Geometry check sheet. Reference: the model listing, model coordinates, mm. Give positions to 0.01 mm unless a question says otherwise; leave off trailing zeros. Loops run counter-clockwise (first coordinate to the right, second up) from the corner with the lowest first, then second, coordinate; pieces in that order, holes last. Notation, with made-up numbers: (83, -18.5) -> (124, -18.5) arc R25 ccw to (124, 16.5) -> close; hole circle Ø1 at (86, 41). An arc over 180 degrees is marked (long way). One line per item, written item: value. Start each with the question number.
(1) Sectioned sample at C-C, the plane z = -16. Record the cut outline in (x, y).
(2) Scan lines: line 1 along X through (y, z) = (-1.8, -15.5); line 2 along Z through (x, y) = (17, -0.85) (1 decimal); line 3 along X through (y, z) = (-1.05, 24). Record each from-to range of solid material in increasing order. Write a range as from..to.
(3) Sectioned sample at B-B, the plane x = 6.5. Record the cut outline in (y, z) (1 decimal).
(4) Gauge pin test, flat end, axial feed: pin 1 Ø5 at (x, z) = (-14, 20) entering from -Y. Record the tip position at first contact, or that the pin passes through.
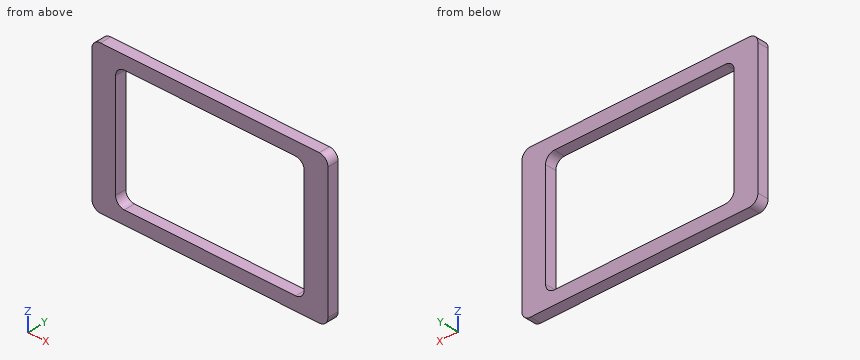
from build123d import *

# Parameters (mm, degrees)
F1_DEPTH = 4


with BuildPart() as f1:
    # F0 (on Front) → F1 (new body)
    with BuildSketch(Plane.XZ):
        with BuildLine():
            Line((0, 26.9875), (-39.7125, 26.9875))
            ThreePointArc((-39.7125, 26.9875), (-41.939886, 26.064886), (-42.8625, 23.8375))
            Line((-42.8625, 23.8375), (-42.8625, 0))
            Line((-42.8625, 0), (-34.25, 0))
            Line((-34.25, 0), (-34.25, 18.95))
            ThreePointArc((-34.25, 18.95), (-33.320064, 21.195064), (-31.075, 22.125))
            Line((-31.075, 22.125), (0, 22.125))
            Line((0, 22.125), (0, 26.9875))
        make_face()
        with BuildLine():
            Line((39.7125, 26.9875), (0, 26.9875))
            Line((0, 26.9875), (0, 22.125))
            Line((0, 22.125), (31.075, 22.125))
            ThreePointArc((31.075, 22.125), (33.320064, 21.195064), (34.25, 18.95))
            Line((34.25, 18.95), (34.25, -18.95))
            ThreePointArc((34.25, -18.95), (33.320064, -21.195064), (31.075, -22.125))
            Line((31.075, -22.125), (-31.075, -22.125))
            ThreePointArc((-31.075, -22.125), (-33.320064, -21.195064), (-34.25, -18.95))
            Line((-34.25, -18.95), (-34.25, 0))
            Line((-34.25, 0), (-42.8625, 0))
            Line((-42.8625, 0), (-42.8625, -23.8375))
            ThreePointArc((-42.8625, -23.8375), (-41.939886, -26.064886), (-39.7125, -26.9875))
            Line((-39.7125, -26.9875), (39.7125, -26.9875))
            ThreePointArc((39.7125, -26.9875), (41.939886, -26.064886), (42.8625, -23.8375))
            Line((42.8625, -23.8375), (42.8625, 23.8375))
            ThreePointArc((42.8625, 23.8375), (41.939886, 26.064886), (39.7125, 26.9875))
        make_face()
    extrude(amount=F1_DEPTH)


solid = f1.part
Calculated:
1. outline: (-42.86, -4) -> (-34.25, -4) -> (-34.25, 0) -> (-42.86, 0) -> close; (34.25, -4) -> (42.86, -4) -> (42.86, 0) -> (34.25, 0) -> close
2. line 1: x = -42.86..-34.25, 34.25..42.86
2. line 2: z = -27..-22.1, 22.1..27
2. line 3: x = -42.86..42.86
3. outline: (-4, -27) -> (0, -27) -> (0, -22.1) -> (-4, -22.1) -> close; (-4, 22.1) -> (0, 22.1) -> (0, 27) -> (-4, 27) -> close
4. pin 1: stops at y = -4
